Check sheet for the modelled part. Datum: model origin and axes. Units: mm. A direction names the side the tool comes from. Coordinates: 2 decimals unless noted, no trailing zeros. Loops run counter-clockwise (first coordinate to the right, second up) from the corner with the lowest first, then second, coordinate; pieces in that order, holes last. Notation, with made-up numbers: (-32, 18) -> (-11, 18) arc R32 ccw to (-11, 50) -> close; hole circle Ø5 at (-14.5, 4). An arc over 180 degrees is marked (long way). Use CSV: the item, a comma, the result in double quotes.
```python
from build123d import *

# Parameters (mm, degrees)
BASE_FLANGE1_DEPTH = 374.65
SKETCH2_R          = 2.45745
CUT_EXTRUDE1_DEPTH = 3.175
SKETCH4_R          = 2.45745
CUT_EXTRUDE2_DEPTH = 3.175
FILLET1_R          = 3.175


# Sheet-metal steps are written as plain solids
with BuildPart() as part:
    # Sketch1 → Base-Flange1 (new body)
    with BuildSketch(Plane(origin=(0, 0, 0), x_dir=(1, 0, 0), z_dir=(0, 1, 0))):
        with BuildLine():
            Line((60.81522, 25.4), (60.81522, 6.35))
            ThreePointArc((60.81522, 6.35), (58.955348061, 1.859871939), (54.46522, 0))
            Line((54.46522, 0), (3.666174209, 0))
            ThreePointArc((3.666174209, 0), (0.491174209, 0.850738686), (-1.833087105, 3.175))
            Line((-1.833087105, 3.175), (-27.23261, 47.168264143))
            ThreePointArc((-27.23261, 47.168264143), (-27.866977683, 51.986765079), (-24.908348686, 55.842525457))
            Line((-24.908348686, 55.842525457), (-8.410564744, 65.367525457))
            Line((-8.410564744, 65.367525457), (-6.823064744, 62.6178948))
            Line((-6.823064744, 62.6178948), (-23.320848686, 53.0928948))
            ThreePointArc((-23.320848686, 53.0928948), (-24.800163184, 51.165014611), (-24.482979343, 48.755764143))
            Line((-24.482979343, 48.755764143), (0.916543552, 4.7625))
            ThreePointArc((0.916543552, 4.7625), (2.078674209, 3.600369343), (3.666174209, 3.175))
            Line((3.666174209, 3.175), (54.46522, 3.175))
            ThreePointArc((54.46522, 3.175), (56.71028403, 4.10493597), (57.64022, 6.35))
            Line((57.64022, 6.35), (57.64022, 25.4))
            Line((57.64022, 25.4), (60.81522, 25.4))
        make_face()
    extrude(amount=BASE_FLANGE1_DEPTH)

    # Sketch2 → Cut-Extrude1 (cut)
    with BuildSketch(Plane.XY):
        with Locations((16.366174209, 361.95)):
            Circle(SKETCH2_R)
        with Locations((16.366174209, 336.55)):
            Circle(SKETCH2_R)
        with Locations((41.766174209, 336.55)):
            Circle(SKETCH2_R)
        with Locations((41.766174209, 361.95)):
            Circle(SKETCH2_R)
        with Locations(Location((41.766174209, 12.7, 0), (0, 0, 180))):
            Circle(SKETCH2_R)
        with Locations(Location((16.366174209, 12.7, 0), (0, 0, 180))):
            Circle(SKETCH2_R)
        with Locations(Location((41.766174209, 38.1, 0), (0, 0, 180))):
            Circle(SKETCH2_R)
        with Locations(Location((16.366174209, 38.1, 0), (0, 0, 180))):
            Circle(SKETCH2_R)
    cut_extrude1 = extrude(amount=-CUT_EXTRUDE1_DEPTH, mode=Mode.SUBTRACT)

    # Sketch4 → Cut-Extrude2 (cut)
    with BuildSketch(Plane(origin=(60.81522, 0, 0), x_dir=(0, 0, -1), z_dir=(1, 0, 0))):
        with Locations((15.875, 361.95)):
            Circle(SKETCH4_R)
        with Locations(Location((15.875, 12.7, 0), (0, 0, 180))):
            Circle(SKETCH4_R)
        with Locations((15.875, 187.325)):
            Circle(SKETCH4_R)
    cut_extrude2 = extrude(amount=-CUT_EXTRUDE2_DEPTH, mode=Mode.SUBTRACT)

    # Mirror1: Cut-Extrude1, Cut-Extrude2 across plane
    add(cut_extrude1.mirror(Plane(origin=(0, 0, 0), x_dir=(-0.49999999999999795, 0, 0.8660254037844398), z_dir=(-0.8660254037844398, 0, -0.49999999999999795))), mode=Mode.SUBTRACT)
    add(cut_extrude2.mirror(Plane(origin=(0, 0, 0), x_dir=(-0.49999999999999795, 0, 0.8660254037844398), z_dir=(-0.8660254037844398, 0, -0.49999999999999795))), mode=Mode.SUBTRACT)

    # Fillet1
    fillet1_edges = [part.edges().sort_by_distance(p)[0] for p in [
        (-7.616814744, 0, -63.992710128),
        (59.22772, 0, -25.4),
        (-7.616814744, 374.65, -63.992710128),
        (59.22772, 374.65, -25.4),
    ]]
    fillet(fillet1_edges, radius=FILLET1_R)


solid = part.part
```
1) Draft check along X on faces 1 (the flat face through (-14.96, 184.7, -57.92)), 2 (the flat face through (-11.961, 184.702, -27.067)), 3 (the cylindrical face through (-27.885, 184.702, -51.919)). Enter one of: released by +X, released by -X, zero draft, split by the parting line, or undercut.
Answer below:
face 1,"released by +X"
face 2,"undercut"
face 3,"released by -X"
2) Thickness scan on line 1 along X through (y, z) = (361, -1); line 2 along Z through (x, y) = (12.5, 100) (3 decimals); line 3 along X through (y, z) = (38, -2). Record the ranges inside material, lowest first. Write a range as from..to.
Answer below:
line 1,"x = 0.25..14.1, 18.63..39.5, 44.03..57.89"
line 2,"z = -3.175..0"
line 3,"x = -0.96..13.91, 18.82..39.31, 44.22..59.09"
3) Go/stop test with flat-tipped pins: pin 1 Ø2.5 at (x, y) = (59, 241.5) entering from -Z; pin 2 Ø12 at (y, z) = (144, -18.5) entering from -X; pin 3 Ø5.5 at (y, z) = (119.5, -16) entering from -X. Record where each tip stops, or that it passes through.
Answer below:
pin 1,"stops at z = -25.4"
pin 2,"stops at x = -14.15"
pin 3,"stops at x = -10.83"
4) Access from +Z, -Z, +X, -X, +Y, -Y to the whole of each face (thin tool, end or side, straight path). Record for faces 4 (the flat face through (-3, 0, -11)), 5 (the flat face through (57.64, 184.7, -15.7)).
Answer below:
face 4,"+Z, -Z, +X, -X, -Y"
face 5,"-Z, +Y, -Y"
5) Cross-section at B-B on z = -44. Record the boundary of the cut face in (x, y).
Answer below:
outline,"(-25.4, 0) -> (-21.74, 0) -> (-21.74, 374.65) -> (-25.4, 374.65) -> close"
